Design review of the part built by this model. Coordinates are the model's own, in mm. Face numbers are marked on the shaded views. A direction names the side the tool comes from. Give positions to 0.01 mm unless a question says otherwise; leave off trailing zeros. Loops run counter-clockwise (first coordinate to the right, second up) from the corner with the lowest first, then second, coordinate; pieces in that order, holes last.
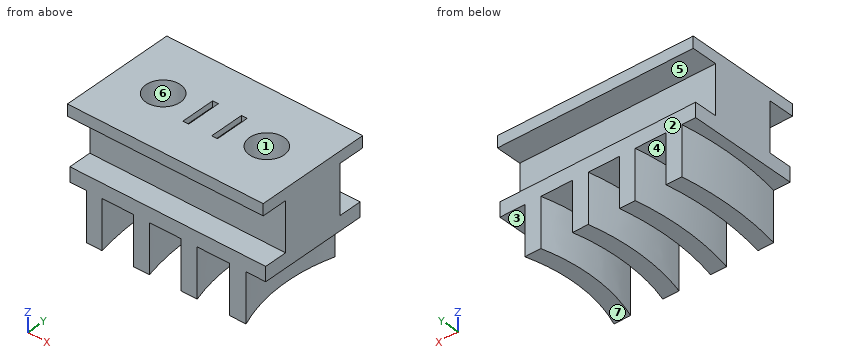
from build123d import *

# Parameters (mm, degrees)
ESQUISSE1_W             = 17
ESQUISSE1_H             = 5.5
BOSS_EXTRU_1_DEPTH      = 5.5
ESQUISSE2_W             = 1.25
ESQUISSE2_H             = 9.5
BOSS_EXTRU_2_DEPTH      = 17
ESQUISSE3_W             = 17
ESQUISSE3_H             = 10
BOSS_EXTRU_3_DEPTH      = 1
ESQUISSE4_R             = 1.5
ENL_V_MAT_EXTRU_1_DEPTH = 3.5
ESQUISSE5_W             = 0.5
ESQUISSE5_H             = 3
ENL_V_MAT_EXTRU_2_DEPTH = 0.5
BOSS_EXTRU_4_DEPTH      = 4.25


with BuildPart() as part:
    # Esquisse1 → Boss.-Extru.1 (new body)
    with BuildSketch(Plane.XY):
        with Locations((20, 0)):
            Rectangle(ESQUISSE1_W, ESQUISSE1_H)
    extrude(amount=-BOSS_EXTRU_1_DEPTH)

    # Esquisse2 → Boss.-Extru.2 (add)
    with BuildSketch(Plane(origin=(28.5, 0, 0), x_dir=(0, 0, -1), z_dir=(1, 0, 0))):
        with Locations((4.875, 0)):
            Rectangle(ESQUISSE2_W, ESQUISSE2_H)
    extrude(amount=-BOSS_EXTRU_2_DEPTH)

    # Esquisse3 → Boss.-Extru.3 (add)
    with BuildSketch(Plane.XY):
        with Locations((20, 0)):
            Rectangle(ESQUISSE3_W, ESQUISSE3_H)
    extrude(amount=BOSS_EXTRU_3_DEPTH)

    # Esquisse4 → Enlèv. mat.-Extru.1 (cut)
    with BuildSketch(Plane.XY.offset(1)):
        with Locations((24.5, 0)):
            Circle(ESQUISSE4_R)
        with Locations((15.5, 0)):
            Circle(ESQUISSE4_R)
    extrude(amount=-ENL_V_MAT_EXTRU_1_DEPTH, mode=Mode.SUBTRACT)

    # Esquisse5 → Enlèv. mat.-Extru.2 (cut)
    with BuildSketch(Plane.XY.offset(1)):
        with Locations((21.25, 0)):
            Rectangle(ESQUISSE5_W, ESQUISSE5_H)
        with Locations((18.75, 0)):
            Rectangle(ESQUISSE5_W, ESQUISSE5_H)
    extrude(amount=-ENL_V_MAT_EXTRU_2_DEPTH, mode=Mode.SUBTRACT)

    # Esquisse6 → Boss.-Extru.4 (add)
    with BuildSketch(Plane(origin=(0, 0, -5.5), x_dir=(-1, 0, 0), z_dir=(0, 0, -1))):
        with BuildLine():
            Line((-22.552794805, -4.75), (-21.148073426, -4.75))
            add(Edge.make_bspline(
                [(-20.826956456, 4.75), (-20.701976007, 4.166184335), (-20.247306857, 1.445543191), (-20.393909727, -1.7940686), (-21.021282717, -4.308854476), (-21.148073426, -4.75)],
                knots=[0.486029583, 0.486029583, 0.486029583, 0.486029583, 0.487632249, 0.493437395, 0.49468936, 0.49468936, 0.49468936, 0.49468936], degree=3))
            Line((-20.826956456, 4.75), (-22.205629087, 4.75))
            add(Edge.make_bspline(
                [(-22.552794805, -4.75), (-22.373592229, -4.173323429), (-21.728969731, -1.663462019), (-21.607804021, 1.583807787), (-22.070035816, 4.161706415), (-22.205629087, 4.75)],
                knots=[0.248115269, 0.248115269, 0.248115269, 0.248115269, 0.249885808, 0.255690519, 0.257428263, 0.257428263, 0.257428263, 0.257428263], degree=3))
        make_face()
        with BuildLine():
            Line((-24.938721269, 4.75), (-26.33817718, 4.75))
            add(Edge.make_bspline(
                [(-26.797581514, -4.75), (-26.395153508, -3.772148074), (-25.672927447, -1.249795135), (-25.669056389, 2.034035882), (-26.163928672, 4.16779276), (-26.33817718, 4.75)],
                knots=[0.135603088, 0.135603088, 0.135603088, 0.135603088, 0.139596288, 0.145400999, 0.147627485, 0.147627485, 0.147627485, 0.147627485], degree=3))
            Line((-26.797581514, -4.75), (-25.352622939, -4.75))
            add(Edge.make_bspline(
                [(-24.938721269, 4.75), (-24.790737954, 4.205700458), (-24.308623009, 1.965116283), (-24.333265983, -1.304768064), (-25.024589159, -3.86460469), (-25.352622939, -4.75)],
                knots=[0.596036757, 0.596036757, 0.596036757, 0.596036757, 0.597930019, 0.603735165, 0.606985384, 0.606985384, 0.606985384, 0.606985384], degree=3))
        make_face()
        with BuildLine():
            Line((-18.401930877, -4.75), (-17.0169294, -4.75))
            add(Edge.make_bspline(
                [(-16.754018342, 4.75), (-16.622548676, 4.006332525), (-16.215434289, 0.825617368), (-16.46223045, -2.389104753), (-17.0169294, -4.75)],
                knots=[0.375646512, 0.375646512, 0.375646512, 0.375646512, 0.377334478, 0.382815018, 0.382815018, 0.382815018, 0.382815018], degree=3))
            Line((-16.754018342, 4.75), (-18.122057744, 4.75))
            add(Edge.make_bspline(
                [(-18.401930877, -4.75), (-18.393480034, -4.716238825), (-17.802884316, -2.332718806), (-17.554252699, 0.889694687), (-17.988042673, 4.036223412), (-18.122057744, 4.75)],
                knots=[0.360091869, 0.360091869, 0.360091869, 0.360091869, 0.360175327, 0.365980039, 0.367700208, 0.367700208, 0.367700208, 0.367700208], degree=3))
        make_face()
        with BuildLine():
            Line((-12.702642178, 4.75), (-14.064547598, 4.75))
            add(Edge.make_bspline(
                [(-14.300001857, -4.75), (-13.846890026, -2.590707185), (-13.586316634, 0.605300957), (-13.912106186, 3.788517123), (-14.064547598, 4.75)],
                knots=[0.471792726, 0.471792726, 0.471792726, 0.471792726, 0.476269559, 0.478227562, 0.478227562, 0.478227562, 0.478227562], degree=3))
            Line((-14.300001857, -4.75), (-12.926181075, -4.75))
            add(Edge.make_bspline(
                [(-12.702642178, 4.75), (-12.548150742, 3.724600153), (-12.249496767, 0.541531469), (-12.507778318, -2.649137977), (-12.926181075, -4.75)],
                knots=[0.265051802, 0.265051802, 0.265051802, 0.265051802, 0.267036708, 0.271169831, 0.271169831, 0.271169831, 0.271169831], degree=3))
        make_face()
    extrude(amount=BOSS_EXTRU_4_DEPTH)


solid = part.part
Q1. Take a section at D-D (x = 27.75). Give the boundary of the cut face in (y, z).
Results:
outline: (-5, 0) - (-2.75, 0) - (-2.75, -4.25) - (-4.75, -4.25) - (-4.75, -5.5) - (4.75, -5.5) - (4.75, -4.25) - (2.75, -4.25) - (2.75, 0) - (5, 0) - (5, 1) - (-5, 1) - close
Q2. Take a section at A-A (z = -1.5). Give the boundary of the cut face in (x, y).
Results:
outline: (11.5, -2.75) - (28.5, -2.75) - (28.5, 2.75) - (11.5, 2.75) - close; hole circle Ø3 at (15.5, 0); hole circle Ø3 at (24.5, 0)
Q3. Wall thickness on line 1 (X direction, y = 0.75, z = -8.5); line 2 (Y direction, x = 15.5, z = -1.35); line 3 (Z direction, x = 16.75, y = 4): over which ranges is each line inside the solid? List them lowest first.
Results:
line 1: x = 12.39 to 13.74, 16.39 to 17.74, 20.39 to 21.74, 24.39 to 25.74
line 2: y = -2.75 to -1.5, 1.5 to 2.75
line 3: z = -9.75 to -4.25, 0 to 1
Q4. Insertion check: pin 1 (5 mm diameter, centred on x = 26, y = -1.5, fed in from -Z); pin 2 (2 mm diameter, centred on x = 21, z = -2.5, fed in from -Y); pin 3 (1.8 mm diameter, centred on x = 23.5, y = -1, fed in from -Z); pin 4 (5 mm diameter, centred on x = 17, z = -3.5, fed in from -Y). Each pin has a flat end and moves straight along its axis. Give the tip position at first contact, or say it passes through.
Results:
pin 1: stops at z = -9.75
pin 2: stops at y = -2.75
pin 3: stops at z = -5.5
pin 4: stops at y = -4.75
Q5. Draft analysis for pull direction Z (two halves, no side actions). For the marked faces 5, 6 and 7, state which applies: pulls with the +Z half, pulls with the -Z half, needs draft (parallel to the pull), parting line crosses it, or undercut.
Results:
face 5: undercut
face 6: needs draft
face 7: pulls with the -Z half
Q6. Tool access review of the marked faces 1, 2, 3 and 4: name each direction out of +Z, -Z, +X, -X, +Y, -Y from which nothing blocks a thin tool from reaching the whole face with its end or side.
Results:
face 1: +Z
face 2: -Z, +X, -X, +Y
face 3: -Z, +X
face 4: -Z
Q7. Take a section at B-B (x = 17.5). Give the boundary of the cut face in (y, z).
Results:
outline: (-5, 0) - (-2.75, 0) - (-2.75, -4.25) - (-4.75, -4.25) - (-4.75, -9.75) - (4.75, -9.75) - (4.75, -4.25) - (2.75, -4.25) - (2.75, 0) - (5, 0) - (5, 1) - (-5, 1) - close
Q8. Take a section at C-C (z = -6.25). Give the number of separate pieces and of enclosed holes in the cut face, plus the area to 3 significant figures.
Results:
separate pieces: 4
enclosed holes: 0
area: 51.7 mm2
